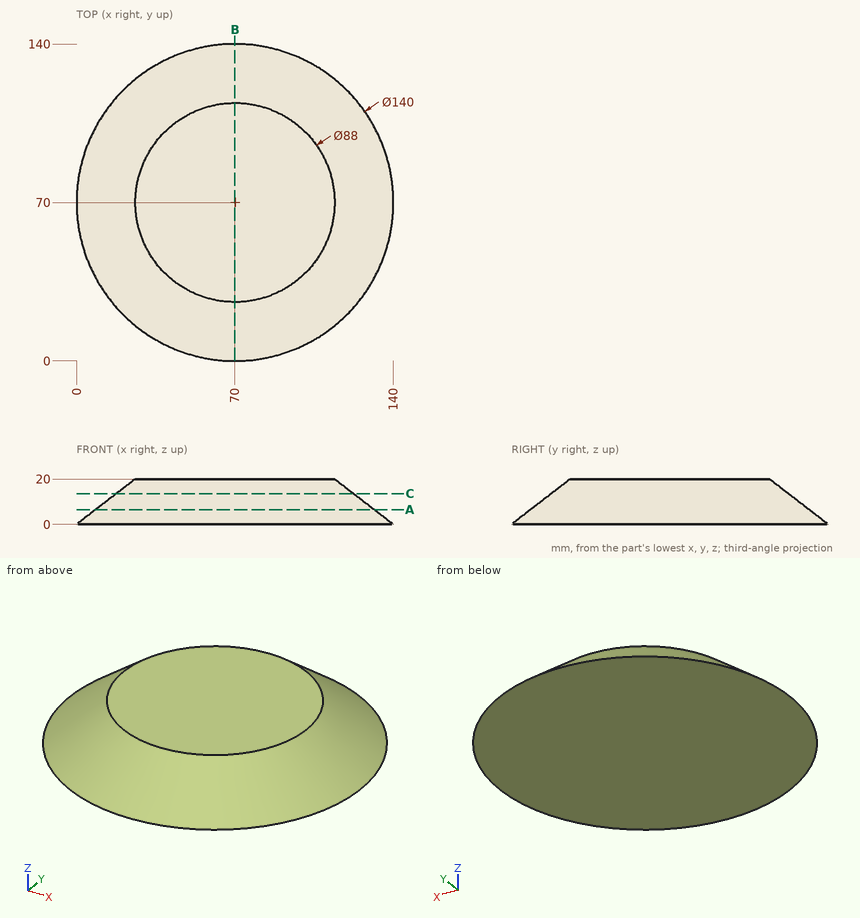
Can you work these out from the drawing? Everything is in mm from the part's minimum corner. Round coordinates to 2 decimals unless told otherwise and drop trailing zeros. Order: outer loops, then holes, each group sorted by start corner. A loop starts at its lowest first (then second) coordinate and runs counter-clockwise, first axis right, second up. Notation, with made-up numbers: (11, -5) -> (54, -5) arc R29 cw to (54, 25) -> close; hole circle Ø5 at (35, 11.25). An arc over 180 degrees is marked (long way). Use CSV: the item, a comma, the result in double quotes.
1. I need wall thicknesses on line 1 along Y through (x, z) = (104, 11.75); line 2 along X through (y, z) = (111.5, 16.5); line 3 along Z through (x, y) = (114.5, 67.5). Which ranges of each line are inside material? Lowest first, please.
Recorded:
line 1,"y = 27.12 to 112.88"
line 2,"x = 44.8 to 95.2"
line 3,"z = 0 to 19.56"
2. I want a section at A-A on z = 6.5. List the corners of the cut face in (x, y) for me, and give its area (3 significant figures).
Recorded:
outline,"circle Ø123.1 at (70, 70)"
area,"11,900 mm2"
3. I want a section at C-C on z = 13.5. List the corners of the cut face in (x, y) for me, and give its area (3 significant figures).
Recorded:
outline,"circle Ø104.9 at (70, 70)"
area,"8,640 mm2"
4. I want a section at B-B on x = 70. List the corners of the cut face in (y, z) for me.
Recorded:
outline,"(0, 0) -> (140, 0) -> (114, 20) -> (26, 20) -> close"
5. I'm going to push flat-ended pins straight in: P1, Ø8, axis at x = 32.5, z = 17.5, coming from the +Y side; P2, Ø5, axis at y = 46.5, z = 16, coming from the -X side; P3, Ø2, axis at x = 58.5, z = 16, coming from the -Y side; P4, Ø4, axis at x = 122, y = 20, coming from the +Z side. Where does each tip first touch, or does it pass through?
Recorded:
P1,"stops at y = 107.66"
P2,"stops at x = 22.91"
P3,"stops at y = 20.81"
P4,"passes through"
